Here's how the part is built. I have some questions about the finished solid (model axes, mm). Face numbers are marked on the shaded views. A direction names the side the tool comes from. Give positions to 0.01 mm unless a question says otherwise; leave off trailing zeros. Write each loop counter-clockwise with the first axis right and the second up, starting at its lowest first coordinate (ties: lowest second). Pieces come first, ordered by that corner, then holes. Notation, with made-up numbers: (20, 4.25) -> (37, 4.25) arc R17 ccw to (37, 28.25) -> close; hole circle Ø6 at (52, -12). An arc over 180 degrees is marked (long way). Use one line per item in the form item = value.
```python
from build123d import *

# Parameters (mm, degrees)
SKETCH1_W           = 22
SKETCH1_H           = 50
BOSS_EXTRUDE1_DEPTH = 60
SKETCH2_R           = 4.1
CUT_EXTRUDE1_DEPTH  = 23
SKETCH4_R           = 9
CUT_EXTRUDE2_DEPTH  = 61
SKETCH5_W           = 22
SKETCH5_H           = 3.3
SKETCH5_H_2         = 7
CUT_EXTRUDE3_DEPTH  = 13


with BuildPart() as part:
    # Sketch1 → Boss-Extrude1 (new body)
    with BuildSketch(Plane(origin=(0, 0, 0), x_dir=(1, 0, 0), z_dir=(0, 1, 0))):
        Rectangle(SKETCH1_W, SKETCH1_H)
    extrude(amount=BOSS_EXTRUDE1_DEPTH)

    # Sketch2 → Cut-Extrude1 (cut, through all)
    with BuildSketch(Plane(origin=(11, 0, 0), x_dir=(0, 0, -1), z_dir=(1, 0, 0))):
        with Locations((-2, 51)):
            Circle(SKETCH2_R)
        with Locations((-2, 9)):
            Circle(SKETCH2_R)
    extrude(amount=-CUT_EXTRUDE1_DEPTH, mode=Mode.SUBTRACT)

    # Sketch4 → Cut-Extrude2 (cut, through all)
    with BuildSketch(Plane(origin=(0, 60, 0), x_dir=(1, 0, 0), z_dir=(0, 1, 0))):
        with Locations((0, 18)):
            Circle(SKETCH4_R)
    extrude(amount=-CUT_EXTRUDE2_DEPTH, mode=Mode.SUBTRACT)

    # Sketch5 → Cut-Extrude3 (cut)
    with BuildSketch(Plane.XY.offset(25)):
        with Locations((0, 40.35)):
            Rectangle(SKETCH5_W, SKETCH5_H)
        with Locations((0, 20.5)):
            Rectangle(SKETCH5_W, SKETCH5_H_2)
    extrude(amount=-CUT_EXTRUDE3_DEPTH, mode=Mode.SUBTRACT)


solid = part.part
```
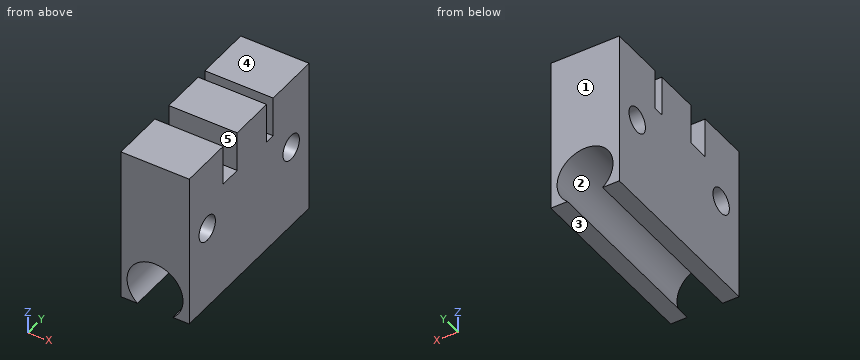
Q1. If I drill on line 1 along Y through (x, z) = (0.75, 2); line 2 along X through (y, z) = (18, -18); line 3 along Z through (x, y) = (0, 38), over which ranges is the centre line in solid material (lowest first)? Write a range as from..to.
Result set:
line_1 = 0..4.9, 13.1..46.9, 55.1..60
line_2 = -11..-9, 9..11
line_3 = -9..25
Q2. I want a section at C-C, the plane x = 0. Write out the boundary of the cut face in (y, z), and give its area (3 significant figures).
Result set:
outline = (0, -9) -> (60, -9) -> (60, 25) -> (42, 25) -> (42, 12) -> (38.7, 12) -> (38.7, 25) -> (24, 25) -> (24, 12) -> (17, 12) -> (17, 25) -> (0, 25) -> close; hole circle Ø8.2 at (9, 2); hole circle Ø8.2 at (51, 2)
area = 1,800 mm2
Q3. Which directions (+Z, -Z, +X, -X, +Y, -Y) give clear straight access to the entire face, cutting with the end or side of a thin tool? Please do the marked faces 4 and 5.
Result set:
face_4 = +Z, +X, -X, +Y, -Y
face_5 = +Z, +X, -X
Q4. If we mould it in two halves opening along Z, with no side actions, what happens to the marked faces 1, 2 and 3? For each: +Z half, -Z half, draft (parallel to the pull), parting line (faces both ways), or undercut.
Result set:
face_1 = draft
face_2 = undercut
face_3 = -Z half
Q5. I want a section at A-A, the plane z = 2. Write out the boundary of the cut face in (x, y), and give its area (3 significant figures).
Result set:
outline = (-11, 0) -> (11, 0) -> (11, 4.9) -> (-11, 4.9) -> close; (-11, 13.1) -> (11, 13.1) -> (11, 46.9) -> (-11, 46.9) -> close; (-11, 55.1) -> (11, 55.1) -> (11, 60) -> (-11, 60) -> close
area = 959 mm2
Q6. Will these pins go through, and if not, where does the flat tip stop? pin 1 Ø2 at (x, y) = (-4, 22.5) entering from +Z; pin 2 Ø11 at (x, z) = (0, -18) entering from -Y.
Result set:
pin_1 = 12
pin_2 = through
Q7. I want a section at B-B, the plane y = 9. Write out the boundary of the cut face in (x, z), and give its area (3 significant figures).
Result set:
outline = (-11, -25) -> (-5.66, -25) arc R9 cw (long way) to (5.66, -25) -> (11, -25) -> (11, -2.1) -> (-11, -2.1) -> close; (-11, 6.1) -> (11, 6.1) -> (11, 25) -> (-11, 25) -> close
area = 681 mm2
Q8. I want a section at D-D, the plane x = -7.5. Write out the boundary of the cut face in (y, z).
Result set:
outline = (0, -25) -> (60, -25) -> (60, -22.97) -> (0, -22.97) -> close; (0, -13.03) -> (60, -13.03) -> (60, 25) -> (42, 25) -> (42, 12) -> (38.7, 12) -> (38.7, 25) -> (24, 25) -> (24, 12) -> (17, 12) -> (17, 25) -> (0, 25) -> close; hole circle Ø8.2 at (9, 2); hole circle Ø8.2 at (51, 2)
